The model under review builds one solid part; all positions refer to its coordinate system, in mm. Round coordinates to 2 decimals unless told otherwise and drop trailing zeros. Order: outer loops, then holes, each group sorted by start corner. A loop starts at its lowest first (then second) coordinate and runs counter-clockwise, first axis right, second up. Notation, with made-up numbers: (-36, 25) -> (11, 25) arc R20 cw to (11, 62) -> close; hole circle Ø3 at (55, 37.25). An arc over 180 degrees is marked (long way). Use a Markdown table: item, result. Add a question column.
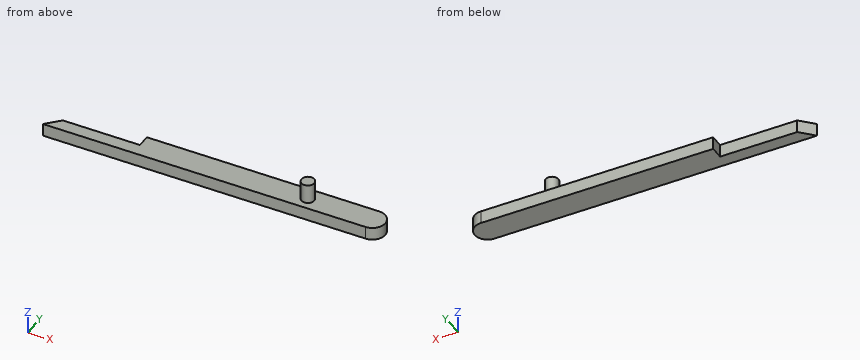
```python
from build123d import *

# Parameters (mm, degrees)
SKETCH1_R           = 10
BOSS_EXTRUDE1_DEPTH = 20
SKETCH1_2_R         = 10
BOSS_EXTRUDE2_DEPTH = 50


with BuildPart() as part:
    # Sketch1 → Boss-Extrude1 (new body)
    with BuildSketch(Plane.XY):
        with BuildLine():
            Line((-229.914228229, 0), (-110.283225042, 0))
            Line((-110.283225042, 0), (-110.283225042, 20))
            Line((-110.283225042, 20), (250, 20))
            ThreePointArc((250, 20), (270, 0), (250, -20))
            Line((250, -20), (-250, -20))
            Line((-250, -20), (-229.914228229, 0))
        make_face()
        with Locations((150, 0)):
            Circle(SKETCH1_R, mode=Mode.SUBTRACT)
    extrude(amount=BOSS_EXTRUDE1_DEPTH)

    # Sketch1<2> → Boss-Extrude2 (add)
    with BuildSketch(Plane.XY):
        with Locations((150, 0)):
            Circle(SKETCH1_2_R)
    extrude(amount=BOSS_EXTRUDE2_DEPTH)


solid = part.part
```
Q1. Add section A-A, the plane z = 15.5. Give the boundary of the cut face in (x, y), then the cut area to 3 significant figures.
Q2. Add section B-B, the plane x = -144.5. Give the boundary of the cut face in (y, z).
Q3. To check wall thickness, follow line 1 along X through (y, z) = (2, 18); line 2 along Z through (x, y) = (13, 7); line 3 along Y through (x, z) = (-152, 10.5). State the ranges of each line that lie inside material, in increasing order.
Q4. Add section C-C, the plane y = -15.5. Give the boundary of the cut face in (x, z), then the cut area to 3 significant figures.
Q5. For pin 1 (12 mm diameter, centred on x = 11, y = 4, fed in from +Z); pin 2 (16 mm diameter, centred on x = -199.5, z = 11, fed in from +Y); pin 3 (3 mm diameter, centred on y = -9.5, z = 44.5, fed in from -X), all flat-tipped, find the tip position at first contact; note any pin that passes through.
Return value:
| question | item | result |
|---|---|---|
| 1 | outline | (-250, -20) -> (250, -20) arc R20 ccw to (250, 20) -> (-110.28, 20) -> (-110.28, 0) -> (-229.91, 0) -> close |
| 1 | area | 17,600 mm² |
| 2 | outline | (-20, 0) -> (0, 0) -> (0, 20) -> (-20, 20) -> close |
| 3 | line 1 | -110.28 to 269.9 |
| 3 | line 2 | 0 to 20 |
| 3 | line 3 | -20 to 0 |
| 4 | outline | (-245.48, 0) -> (262.64, 0) -> (262.64, 20) -> (-245.48, 20) -> close |
| 4 | area | 10,200 mm² |
| 5 | pin 1 | z = 20 |
| 5 | pin 2 | y = 0 |
| 5 | pin 3 | x = 144 |
